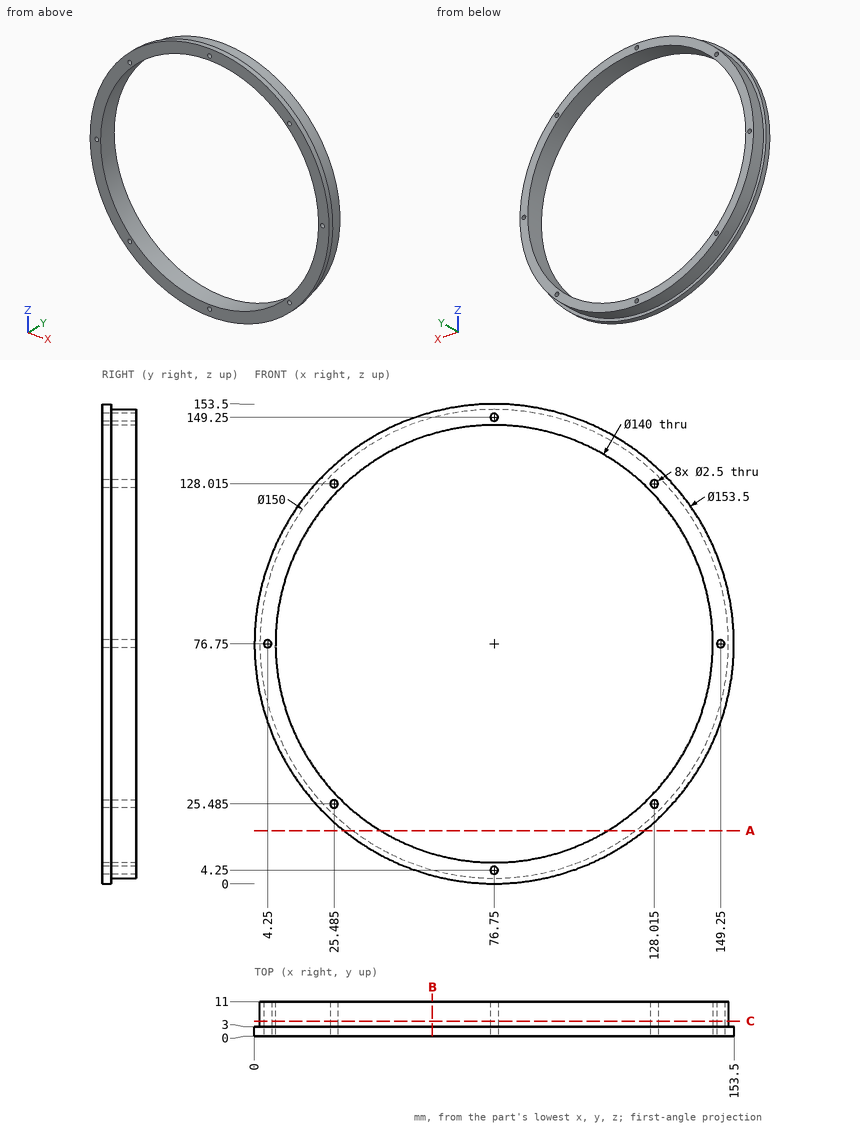
Could you check a few things on this drawing? It's one solid part, dimensions in mm from its lowest x, y, z. Coordinates: 2 decimals unless noted, no trailing zeros. Order: outer loops, then holes, each group sorted by start corner. A loop starts at its lowest first (then second) coordinate and runs counter-clockwise, first axis right, second up. Notation, with made-up numbers: (83.25, 28.25) - (136.25, 28.25) arc R16 ccw to (136.25, 42.25) - close; hole circle Ø8 at (6.25, -15.75). An arc over 180 degrees is marked (long way). Answer as a JSON object with one key per item and string values. Group by question number.
Q1. Imagine slicing it at C-C (y = 4.75). Give the number of separate pieces and of enclosed holes in the cut face, and give its area (3 significant figures).
Q2. I need wall thicknesses on line 1 (X direction, y = 6.25, z = 76.75); line 2 (Z direction, x = 33.5, y = 9.5); line 3 (Z direction, x = 36.5, y = 7) (1 decimal). Which ranges of each line are inside material? Lowest first, please. Write a range as from..to.
Q3. Imagine slicing it at B-B (x = 57). Please give me the cut outline in (y, z) (1 decimal).
Q4. Imagine slicing it at A-A (z = 17). Please give me the cut outline in (x, y).
Q5. Will these pins go through, and if not, where does the flat tip stop? P1, Ø3, axis at x = 128.02, z = 25.48, coming from the -Y side; P2, Ø1, axis at x = 22, y = 8, coming from the -Z side; P3, Ø1, axis at y = 5, z = 116.5, coming from the -X side.
Determined:
{
 "1": {"separate pieces": "1", "enclosed holes": "9", "area": "2,240 mm2"},
 "2": {"line 1": "x = 1.75..3, 5.5..6.75, 146.75..148, 150.5..151.75", "line 2": "z = 15.48..21.71, 131.79..138.02", "line 3": "z = 13.5..19.5, 134..140"},
 "3": {"outline": "(0, 2.6) - (3, 2.6) - (3, 4.4) - (11, 4.4) - (11, 9.6) - (0, 9.6) - close; (0, 143.9) - (11, 143.9) - (11, 149.1) - (3, 149.1) - (3, 150.9) - (0, 150.9) - close"},
 "4": {"outline": "(28.58, 0) - (40.28, 0) - (40.28, 11) - (31.42, 11) - (31.42, 3) - (28.58, 3) - close; (113.22, 0) - (124.92, 0) - (124.92, 3) - (122.08, 3) - (122.08, 11) - (113.22, 11) - close"},
 "5": {"P1": "stops at y = 0", "P2": "stops at z = 24.96", "P3": "stops at x = 12.84"}
}
